Study the drawing (mm; zero at the part's minimum x, y, z) and answer. A direction names the side the tool comes from. Coordinates: 2 decimals unless noted, no trailing zeros. Order: outer loops, then holes, each group sorted by start corner. A loop starts at its lowest first (then second) coordinate and runs counter-clockwise, first axis right, second up. Notation, with made-up numbers: M -16,-18 L 32,-18 A36 ccw 32,16 Z; hole C -38.75,-33 d6. An arc over 180 degrees is marked long. Use a Markdown table: item, result. Add a question column.
1) This flat-tipped pin is pushed along its axis until it touches: pin 1 Ø2.5 at (y, z) = (5.5, 5) entering from +X. Where does it stop, or does it pass through?
2) The mould has two halves that part along Z. Classify the marked faces 1, 2 and 3: released by +Z, released by -Z, zero draft, split by the parting line, or undercut.
3) For the marked faces 4 and 5, determine the directions among +Z, -Z, +X, -X, +Y, -Y from which every point of the face is accessible in a straight line to the end or side of a thin tool.
4) Find section D-D on x = 1. Write down the section's boundary in (y, z), plus the area to 3 significant figures.
5) Find section C-C on x = 3.7. Write down the section's boundary in (y, z).
6) Find the intervals of material crossed by probe 1 along Y at (x, z) = (2.85, 5); probe 2 along Y at (x, z) = (0.7, 5); probe 3 along X at (y, z) = (5.75, 3.5), in increasing order. Write a range as [from, to].
7) Find section A-A on z = 5. Write down the section's boundary in (x, y), plus the area to 3 significant figures.
8) Find section B-B on y = 5.25. Write down the section's boundary in (x, z).
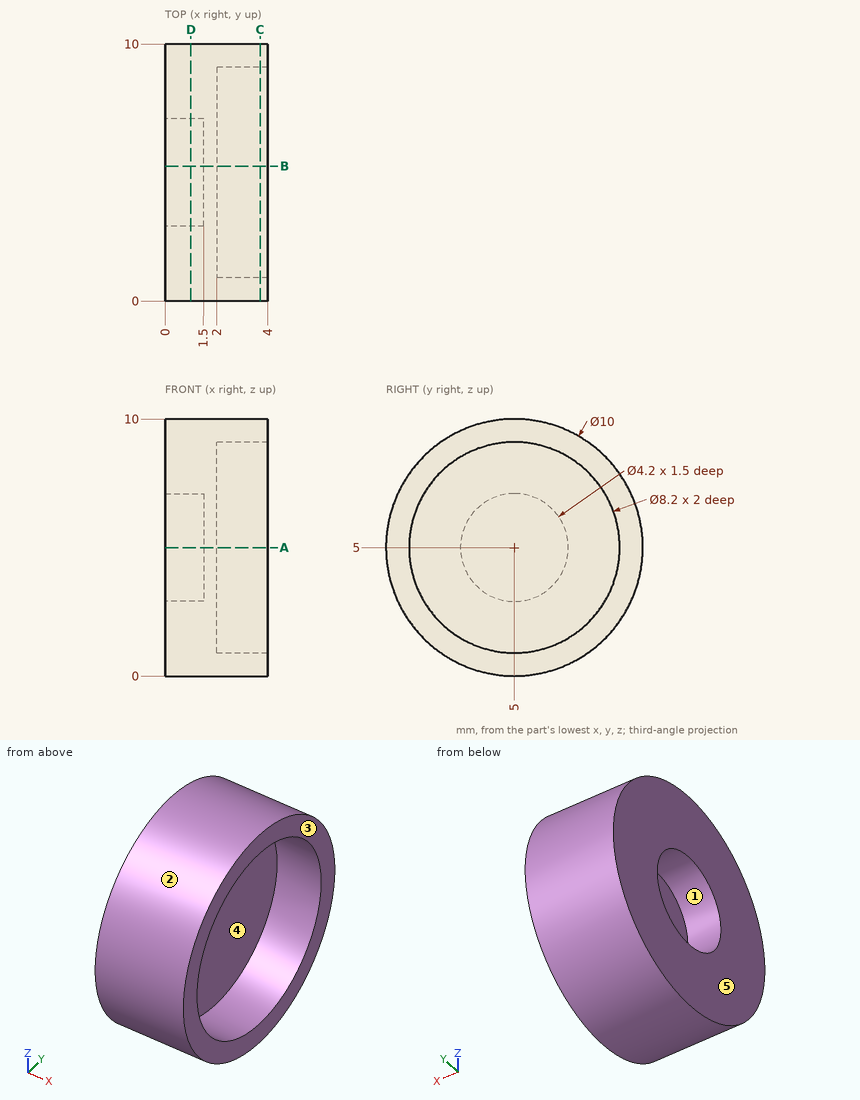
Check result:
| question | item | result |
|---|---|---|
| 1 | pin 1 | stops at x = 2 |
| 2 | face 1 | undercut |
| 2 | face 2 | split by the parting line |
| 2 | face 3 | zero draft |
| 3 | face 4 | +X |
| 3 | face 5 | +Z, -Z, -X, +Y, -Y |
| 4 | outline | C 5,5 d10; hole C 5,5 d4.2 |
| 4 | area | 64.7 mm2 |
| 5 | outline | C 5,5 d10; hole C 5,5 d8.2 |
| 6 | probe 1 | y = [0, 0.9], [9.1, 10] |
| 6 | probe 2 | y = [0, 2.9], [7.1, 10] |
| 6 | probe 3 | x = [1.5, 2] |
| 7 | outline | M 0,0 L 4,0 L 4,0.9 L 2,0.9 L 2,9.1 L 4,9.1 L 4,10 L 0,10 L 0,7.1 L 1.5,7.1 L 1.5,2.9 L 0,2.9 Z |
| 7 | area | 17.3 mm2 |
| 8 | outline | M 0,0.01 L 4,0.01 L 4,0.91 L 2,0.91 L 2,9.09 L 4,9.09 L 4,9.99 L 0,9.99 L 0,7.09 L 1.5,7.09 L 1.5,2.91 L 0,2.91 Z |
